Autodesk Inventor part; units mm, degrees
ref_plane "YZ Plane" through (0, 0, 0) normal (1, 0, 0) x (0, 1, 0)
ref_plane "XZ Plane" through (0, 0, 0) normal (0, 1, 0) x (-1, 0, 0)
ref_plane "XY Plane" through (0, 0, 0) normal (0, 0, 1) x (1, 0, 0)
sketch "Sketch1" plane through (0, 0, 0) normal (0, 0, 1) x (1, 0, 0)
  line L0 (-56, -58) -> (56, -58)
  line L1 (56, -58) -> (56, 58)
  line L2 (56, 58) -> (-56, 58)
  line L3 (-56, 58) -> (-56, -58)
  line L4 (-56, -58) -> (56, 58) construction
  line L5 (56, -58) -> (-56, 58) construction
  point P0 (0, 0)
  dimension "d0" = 116
  dimension "d1" = 112
extrude "Extrusion1" add sketch "Sketch1" along normal blind 1.6
fillet "Fillet1" radius 2 4 edges at (-56, 58, 0.8) (-56, -58, 0.8) (56, -58, 0.8) (56, 58, 0.8)
sketch "Sketch5" plane through (0, 0, 1.6) normal (0, 0, 1) x (1, 0, 0)
  circle A0 centre (-2, -3) radius 1.6
  circle A1 centre (-6, -44) radius 1.6
  circle A2 centre (40, -53) radius 1.6
  circle A3 centre (51, -42) radius 1.6
  circle A4 centre (51, -12) radius 1.6
  line L0 (56, -56) -> (56, 56) construction
  line L1 (-54, -58) -> (54, -58) construction
  line L2 (0, 81.2) -> (0, -81.2) construction
  line L3 (-78.4, 0) -> (78.4, 0) construction
  circle A5 centre (-40, -53) radius 1.6
  circle A6 centre (-51, -42) radius 1.6
  circle A7 centre (-51, -12) radius 1.6
  circle A8 centre (40, 53) radius 1.6
  circle A9 centre (51, 42) radius 1.6
  circle A10 centre (51, 12) radius 1.6
  line L4 (-54, 58) -> (54, 58) construction
  circle A11 centre (-51, 12) radius 1.6
  circle A12 centre (-51, 42) radius 1.6
  circle A13 centre (-40, 53) radius 1.6
  circle A14 centre (16, 53) radius 1.6
  circle A15 centre (-16, 53) radius 1.6
  point P0 (0, 0)
  point P1 (-56, -56)
  point P2 (-56, 56)
  dimension "d19" = 44
  dimension "d20" = 6
  dimension "d21" = 3
  dimension "d22" = 2
  dimension "d23" = 5
  dimension "d24" = 5
  dimension "d25" = 5
  dimension "d27" = 3.2
  dimension "d28" = 3.2
  dimension "d29" = 3.2
  dimension "d31" = 3.2
  dimension "d32" = 3.2
  dimension "d33" = 16
  dimension "d34" = 16
  dimension "d35" = 12
  dimension "d36" = 3.2
  dimension "d37" = 3.2
  dimension "d38" = 5
  dimension "d39" = 5
  dimension "d40" = 16
  dimension "d41" = 16
extrude "Extrusion4" cut sketch "Sketch5" against normal through all
sketch "OCU_PCB_OUTLINE" plane through (0, 0, 1.6) normal (0, 0, 1) x (1, 0, 0)
  circle A0 centre (18.0683, -23.4912) radius 0.7836
  circle A1 centre (-27.1869, 27.3078) radius 0.7836
  circle A2 centre (18.0683, 27.3078) radius 0.7836
  line L0 (32.6352, -42.846) -> (12.62, -42.846)
  line L1 (32.6352, -42.846) -> (12.62, -42.846)
  arc A3 (32.6352, -42.846) -> (39.7472, -35.734) centre (32.6352, -35.734) ccw
  line L2 (39.7472, -12.62) -> (39.7472, -35.734)
  arc A4 (39.7472, -12.62) -> (32.6352, -5.508) centre (32.6352, -12.62) ccw
  line L3 (12.62, -5.508) -> (32.6352, -5.508)
  arc A5 (12.62, -5.508) -> (5.508, -12.62) centre (12.62, -12.62) ccw
  line L4 (5.508, -35.734) -> (5.508, -12.62)
  arc A6 (5.508, -35.734) -> (12.62, -42.846) centre (12.62, -35.734) ccw
  arc A7 (-16.9126, -36.0388) -> (-5.4826, -24.6088) centre (-16.9126, -24.6088) ccw
  arc A8 (-16.9126, -36.0388) -> (-5.4826, -24.6088) centre (-16.9126, -24.6088) ccw
  line L5 (-5.4826, -21.0528) -> (-5.4826, -24.6088)
  arc A9 (-5.4826, -21.0528) -> (-16.9126, -9.6228) centre (-16.9126, -21.0528) ccw
  line L6 (-28.3426, -9.6228) -> (-16.9126, -9.6228)
  arc A10 (-28.3426, -9.6228) -> (-39.7726, -21.0528) centre (-28.3426, -21.0528) ccw
  line L7 (-39.7726, -24.6088) -> (-39.7726, -21.0528)
  arc A11 (-39.7726, -24.6088) -> (-28.3426, -36.0388) centre (-28.3426, -24.6088) ccw
  line L8 (-16.9126, -36.0388) -> (-28.3426, -36.0388)
  arc A12 (-12.62, 3.508) -> (-5.508, 10.62) centre (-12.62, 10.62) ccw
  arc A13 (-12.62, 3.508) -> (-5.508, 10.62) centre (-12.62, 10.62) ccw
  line L9 (-5.508, 38.179) -> (-5.508, 10.62)
  arc A14 (-5.508, 38.179) -> (-12.62, 45.291) centre (-12.62, 38.179) ccw
  line L10 (-32.6352, 45.291) -> (-12.62, 45.291)
  arc A15 (-32.6352, 45.291) -> (-39.7472, 38.179) centre (-32.6352, 38.179) ccw
  line L11 (-39.7472, 10.62) -> (-39.7472, 38.179)
  arc A16 (-39.7472, 10.62) -> (-32.6352, 3.508) centre (-32.6352, 10.62) ccw
  line L12 (-12.62, 3.508) -> (-32.6352, 3.508)
  arc A17 (5, 10.62) -> (12.62, 3) centre (12.62, 10.62) ccw
  arc A18 (5, 10.62) -> (12.62, 3) centre (12.62, 10.62) ccw
  line L13 (32.6352, 3) -> (12.62, 3)
  arc A19 (32.6352, 3) -> (40.2552, 10.62) centre (32.6352, 10.62) ccw
  line L14 (40.2552, 38.179) -> (40.2552, 10.62)
  arc A20 (40.2552, 38.179) -> (32.6352, 45.799) centre (32.6352, 38.179) ccw
  line L15 (12.62, 45.799) -> (32.6352, 45.799)
  arc A21 (12.62, 45.799) -> (5, 38.179) centre (12.62, 38.179) ccw
  line L16 (5, 10.62) -> (5, 38.179)
  circle A22 centre (-19.8971, -23.4785) radius 0.7836
  circle A23 centre (51, -42) radius 1.6
  circle A24 centre (-51, -42) radius 1.6
  circle A25 centre (-51, 42) radius 1.6
  circle A26 centre (51, 42) radius 1.6
  circle A27 centre (40, 53) radius 1.6
  circle A28 centre (-51, 12) radius 1.6
  circle A29 centre (-40, -53) radius 1.6
  circle A30 centre (40, -53) radius 1.6
  circle A31 centre (51, -12) radius 1.6
  circle A32 centre (-51, -12) radius 1.6
  circle A33 centre (-40, 53) radius 1.6
  circle A34 centre (51, 12) radius 1.6
  circle A35 centre (16, 53) radius 1.6
  circle A36 centre (-2, -3) radius 1.6
  circle A37 centre (-6, -44) radius 1.6
  circle A38 centre (-16, 53) radius 1.6
  arc A39 (56, 56) -> (54, 58) centre (54, 56) ccw
  line L17 (54, 58) -> (-54, 58)
  arc A40 (-54, 58) -> (-56, 56) centre (-54, 56) ccw
  line L18 (-56, 56) -> (-56, -56)
  arc A41 (-56, -56) -> (-54, -58) centre (-54, -56) ccw
  line L19 (-54, -58) -> (54, -58)
  arc A42 (54, -58) -> (56, -56) centre (54, -56) ccw
  line L20 (56, -56) -> (56, 56)
  point P0 (0, 0)
equation "\"d24\" = d23"
equation "\"d25\" = d23"
equation "\"d28\" = d27"
equation "\"d29\" = d27"
equation "\"d31\" = d27"
equation "\"d32\" = d27"
equation "\"d36\" = d27"
equation "\"d37\" = d27"
equation "\"d38\" = d23"
equation "\"d39\" = d23"
equation "\"d40\" = d34"
equation "\"d41\" = d34"
properties part number "OCU_PCB"
Verification items for the finished model (mm, model axes). Coordinates: 2 decimals unless noted, no trailing zeros. Order: outer loops, then holes, each group sorted by start corner. A loop starts at its lowest first (then second) coordinate and runs counter-clockwise, first axis right, second up.
Item 1: Section check A-A, the plane x = -16. Enter the section's corners in (y, z), then the cut area to 3 significant figures.
Filled in:
outline: (-58, 0) - (51.4, 0) - (51.4, 1.6) - (-58, 1.6) - close; (54.6, 0) - (58, 0) - (58, 1.6) - (54.6, 1.6) - close
area: 180 mm2
Item 2: Section check B-B, the plane y = 53. Enter the section's corners in (x, z).
Filled in:
outline: (-56, 0) - (-41.6, 0) - (-41.6, 1.6) - (-56, 1.6) - close; (-38.4, 0) - (-17.6, 0) - (-17.6, 1.6) - (-38.4, 1.6) - close; (-14.4, 0) - (14.4, 0) - (14.4, 1.6) - (-14.4, 1.6) - close; (17.6, 0) - (38.4, 0) - (38.4, 1.6) - (17.6, 1.6) - close; (41.6, 0) - (56, 0) - (56, 1.6) - (41.6, 1.6) - close
Item 3: Section check D-D, the plane y = 12. Enter the section's corners in (x, z).
Filled in:
outline: (-56, 0) - (-52.6, 0) - (-52.6, 1.6) - (-56, 1.6) - close; (-49.4, 0) - (49.4, 0) - (49.4, 1.6) - (-49.4, 1.6) - close; (52.6, 0) - (56, 0) - (56, 1.6) - (52.6, 1.6) - close
Item 4: Section check C-C, the plane x = 51. Enter the section's corners in (y, z), then the cut area to 3 significant figures.
Filled in:
outline: (-58, 0) - (-43.6, 0) - (-43.6, 1.6) - (-58, 1.6) - close; (-40.4, 0) - (-13.6, 0) - (-13.6, 1.6) - (-40.4, 1.6) - close; (-10.4, 0) - (10.4, 0) - (10.4, 1.6) - (-10.4, 1.6) - close; (13.6, 0) - (40.4, 0) - (40.4, 1.6) - (13.6, 1.6) - close; (43.6, 0) - (58, 0) - (58, 1.6) - (43.6, 1.6) - close
area: 165 mm2
Item 5: Release check for a two-part mould opening along Y. For faces 1 (the face through (-39.26, -54.42, 0.81)), 2 (the face through (-1, 1, 0)) record: +Y half, -Y half, draft (parallel to the pull), parting line (faces both ways), or undercut.
Filled in:
face 1: undercut
face 2: draft
Item 6: Material ranges on L1, parallel to Y at x = -40, z = 0.5; L2, parallel to X at y = 43, z = 0.25; L3, parallel to Y at x = 51, z = 0.5, recorded low to high.
Filled in:
L1: y = -58 to -54.6, -51.4 to 51.4, 54.6 to 58
L2: x = -56 to -52.25, -49.75 to 49.75, 52.25 to 56
L3: y = -58 to -43.6, -40.4 to -13.6, -10.4 to 10.4, 13.6 to 40.4, 43.6 to 58
